The listing builds one solid part. Answer for the finished solid, in the listing's coordinates (mm). A direction names the side the tool comes from. Give positions to 0.01 mm unless a question says otherwise; leave off trailing zeros. Write each loop counter-clockwise with the first axis right and the second up, starting at its lowest first coordinate (ties: lowest second). Pieces come first, ordered by that corner, then holes.
```python
from build123d import *

# Parameters (mm, degrees)
SKETCH1_W           = 57
SKETCH1_H           = 38
BOSS_EXTRUDE1_DEPTH = 1.2
SKETCH3_W           = 3.7
SKETCH3_H           = 2.5
SKETCH3_W_2         = 3
SKETCH3_H_2         = 8
SKETCH3_W_3         = 12
BOSS_EXTRUDE2_DEPTH = 2


with BuildPart() as part:
    # Sketch1 → Boss-Extrude1 (new body)
    with BuildSketch(Plane(origin=(0, 0, 0), x_dir=(1, 0, 0), z_dir=(0, 1, 0))):
        with Locations((-1.5, 0)):
            Rectangle(SKETCH1_W, SKETCH1_H)
    extrude(amount=BOSS_EXTRUDE1_DEPTH)

    # Sketch3 → Boss-Extrude2 (add)
    with BuildSketch(Plane(origin=(0, 1.2, 0), x_dir=(1, 0, 0), z_dir=(0, 1, 0))):
        Polygon((-22.7, -16.5), (-27, -16.5), (-27, -10), (-30, -10), (-30, -19), (-22.7, -19), align=None)
        with Locations((-14.85, -17.75)):
            Rectangle(SKETCH3_W, SKETCH3_H)
        with Locations((-28.5, 0)):
            Rectangle(SKETCH3_W_2, SKETCH3_H_2)
        with Locations((-1, -17.75)):
            Rectangle(SKETCH3_W_3, SKETCH3_H)
        Polygon((11, -16.5), (11, -19), (27, -19), (27, -3), (24.5, -3), (24.5, -16.5), align=None)
        Polygon((24.5, 16.5), (24.5, 3), (27, 3), (27, 19), (11, 19), (11, 16.5), align=None)
        Polygon((-30, 10), (-27, 10), (-27, 16.5), (-22.7, 16.5), (-22.7, 19), (-30, 19), align=None)
        with Locations((-1, 17.75)):
            Rectangle(SKETCH3_W_3, SKETCH3_H)
        with Locations((-14.85, 17.75)):
            Rectangle(SKETCH3_W, SKETCH3_H)
    extrude(amount=BOSS_EXTRUDE2_DEPTH)


solid = part.part
```
Item 1: A cutting plane is placed at C-C, the plane x = -2. Give the vertices of the cut face in (y, z).
Conclusion:
outline: (0, -19) - (3.2, -19) - (3.2, -16.5) - (1.2, -16.5) - (1.2, 16.5) - (3.2, 16.5) - (3.2, 19) - (0, 19) - close
Item 2: A cutting plane is placed at A-A, the plane y = 2.5. Count the separate pieces of the cut face and the enclosed holes in it, plus the area to 4 significant figures.
Conclusion:
separate pieces: 9
enclosed holes: 0
area: 325.5 mm2
Item 3: A cutting plane is placed at D-D, the plane z = 1. Give the vertices of the cut face in (x, y).
Conclusion:
outline: (-30, 0) - (27, 0) - (27, 1.2) - (-27, 1.2) - (-27, 3.2) - (-30, 3.2) - close
Item 4: This flat-tipped pin is pushed along its axis until it touches: P1, Ø2, axis at x = -11.5, z = 11, coming from the +Y side. Where does it stop, or does it pass through?
Conclusion:
P1: stops at y = 1.2
Item 5: Which of the six approach directions +Z, -Z, +X, -X, +Y, -Y give full straight-line access (tool end or side, diameter ignored) to faces 4 (the face through (-15, 2, -16.5)), 5 (the face through (11, 2, 18)), 6 (the face through (-28, 2, 10))?
Conclusion:
face 4: +Y
face 5: +Z, -Z, +Y
face 6: -X, +Y
Item 6: Consider probe 1 along X at (y, z) = (2, 12); probe 2 along Z at (x, y) = (-4.5, 1.9); probe 3 along Y at (x, z) = (22, -9). Determine where each line is inside the solid, lowest interval first.
Conclusion:
probe 1: x = -30 to -27, 24.5 to 27
probe 2: z = -19 to -16.5, 16.5 to 19
probe 3: y = 0 to 1.2
Item 7: A cutting plane is placed at B-B, the plane z = -5. Give the vertices of the cut face in (x, y).
Conclusion:
outline: (-30, 0) - (27, 0) - (27, 3.2) - (24.5, 3.2) - (24.5, 1.2) - (-30, 1.2) - close
Item 8: Determine the mould class of faces 1 (the face through (-30, 2, 0)), 2 (the face through (24.5, 2, 10)), 3 (the face through (-29, 2, 4)) for opening direction X: pulls with the +X half, pulls with the -X half, needs draft (parallel to the pull), parting line crosses it, or undercut.
Conclusion:
face 1: pulls with the -X half
face 2: undercut
face 3: needs draft
